Check sheet for the modelled part. Datum: model origin and axes. Units: mm. Round coordinates to 2 decimals unless told otherwise and drop trailing zeros. Loops run counter-clockwise (first coordinate to the right, second up) from the corner with the lowest first, then second, coordinate; pieces in that order, holes last. Notation, with made-up numbers: (2.5, 41.25) - (15.5, 41.25) arc R27 ccw to (15.5, 80.25) - close; hole circle Ø2 at (24.5, 49). An arc over 180 degrees is marked (long way). Answer in a Markdown table with one row per item. Add a question column.
(1) Cross-section at C-C on y = 5. Enter the section's corners in (x, z).
(2) Cross-section at D-D on z = 0.5. Count the separate pieces of the cut face and the enclosed holes in it, then the cut area to 3 significant figures.
(3) Mould release check, pull along Y, two halves, no side actions. Record for faces 1 (the flat face through (3, 3, 1)), 2 (the cylindrical face through (0.1, -8.5, 0.5)), 3 (the cylindrical face through (-0.867, -3.905, 0.507)): +Y half, -Y half, draft (parallel to the pull), parting line (faces both ways), or undercut.
(4) Cross-section at B-B on y = 0. Enter the section's corners in (x, z), then the cut area to 3 significant figures.
(5) Thickness scan on line 1 along X through (y, z) = (6.5, 0.4); line 2 along Y through (x, z) = (0, 0.5); line 3 along X through (y, z) = (-5, 0.1). Record the ranges inside material, lowest first.
(6) Cross-section at A-A on x = 0. Enter the section's corners in (y, z).
from build123d import *

# Parameters (mm, degrees)
F0_R     = 12.5
F0_R_2   = 1
F0_R_3   = 4
F2_R     = 4
F4_DEPTH = 1
F5_R     = 1


with BuildPart() as f3:
    # F3: sweep along a path in F1
    with BuildLine(Plane.XZ) as f3_path:
        Line((0, 0), (0, 1))
    # F0 (on Top) → F3 (sweep)
    with BuildSketch(Plane.XY):
        Circle(F0_R)
        with Locations((-5.6568542495, -5.6568542495)):
            Circle(F0_R_2, mode=Mode.SUBTRACT)
        with Locations((5.6568542495, -5.6568542495)):
            Circle(F0_R_2, mode=Mode.SUBTRACT)
        with Locations((-5.6568542495, 5.6568542495)):
            Circle(F0_R_2, mode=Mode.SUBTRACT)
        Circle(F0_R_3, mode=Mode.SUBTRACT)
        with Locations((5.6568542495, 5.6568542495)):
            Circle(F0_R_2, mode=Mode.SUBTRACT)
    sweep(path=f3_path.line)

    # F2 (on Top) → F4 (cut, through all)
    with BuildSketch(Plane.XY):
        with Locations((0, -12.5)):
            Circle(F2_R)
    extrude(amount=F4_DEPTH, mode=Mode.SUBTRACT)

    # F5
    f5_edges = [f3.edges().sort_by_distance(p)[0] for p in [
        (-3.948468, -11.86, 0.5),
        (3.948468, -11.86, 0.5),
    ]]
    fillet(f5_edges, radius=F5_R)


solid = f3.part
Answers:
| question | item | result |
|---|---|---|
| 1 | outline | (-11.46, 0) - (-6.41, 0) - (-6.41, 1) - (-11.46, 1) - close; (-4.9, 0) - (4.9, 0) - (4.9, 1) - (-4.9, 1) - close; (6.41, 0) - (11.46, 0) - (11.46, 1) - (6.41, 1) - close |
| 2 | separate pieces | 1 |
| 2 | enclosed holes | 5 |
| 2 | area | 404 mm^2 |
| 3 | face 1 | draft |
| 3 | face 2 | -Y half |
| 3 | face 3 | undercut |
| 4 | outline | (-12.5, 0) - (-4, 0) - (-4, 1) - (-12.5, 1) - close; (4, 0) - (12.5, 0) - (12.5, 1) - (4, 1) - close |
| 4 | area | 17.0 mm^2 |
| 5 | line 1 | x = -10.68 to -6.19, -5.12 to 5.12, 6.19 to 10.68 |
| 5 | line 2 | y = -8.5 to -4, 4 to 12.5 |
| 5 | line 3 | x = -11.46 to -6.41, -4.9 to 4.9, 6.41 to 11.46 |
| 6 | outline | (-8.5, 0) - (-4, 0) - (-4, 1) - (-8.5, 1) - close; (4, 0) - (12.5, 0) - (12.5, 1) - (4, 1) - close |
